from build123d import *

# Parameters (mm, degrees)
SKETCH1_W           = 203.2
SKETCH1_H           = 101.6
SKETCH1_R           = 1.27
SKETCH1_R_2         = 7.5184
SKETCH1_R_3         = 2.032
BOSS_EXTRUDE1_DEPTH = 3.175
SKETCH2_W           = 25.908
SKETCH2_H           = 3.175
CUT_EXTRUDE1_DEPTH  = 3.175
SKETCH3_W           = 25.908
SKETCH3_H           = 3.175
CUT_EXTRUDE2_DEPTH  = 3.175
SKETCH5_W           = 25.908
SKETCH5_H           = 3.175
CUT_EXTRUDE3_DEPTH  = 3.175
SKETCH6_W           = 25.908
SKETCH6_H           = 3.175
CUT_EXTRUDE4_DEPTH  = 3.175
SKETCH7_W           = 3.81
SKETCH7_H           = 19.558
CUT_EXTRUDE5_DEPTH  = 3.175


with BuildPart() as part:
    # Sketch1 → Boss-Extrude1 (new body)
    with BuildSketch(Plane(origin=(0, 0, 0), x_dir=(1, 0, 0), z_dir=(0, 1, 0))):
        with Locations((26.275862069, -0.437931034)):
            Rectangle(SKETCH1_W, SKETCH1_H)
        with Locations((120.357219561, 32.709068966)):
            Circle(SKETCH1_R, mode=Mode.SUBTRACT)
        with Locations((120.357219561, 42.869068966)):
            Circle(SKETCH1_R, mode=Mode.SUBTRACT)
        with Locations((-30.609137931, 35.837068966)):
            Circle(SKETCH1_R_2, mode=Mode.SUBTRACT)
        with Locations((-43.709137931, 35.837068966)):
            Circle(SKETCH1_R_3, mode=Mode.SUBTRACT)
        with Locations((-21.859137931, 44.737068966)):
            Circle(SKETCH1_R, mode=Mode.SUBTRACT)
        with Locations((-21.859137931, 26.937068966)):
            Circle(SKETCH1_R, mode=Mode.SUBTRACT)
    extrude(amount=BOSS_EXTRUDE1_DEPTH)

    # Sketch2 → Cut-Extrude1 (cut)
    with BuildSketch(Plane(origin=(0, 0, -50.362068966), x_dir=(-1, 0, 0), z_dir=(0, 0, -1))):
        with Locations((-89.775862069, 1.5875)):
            Rectangle(SKETCH2_W, SKETCH2_H)
        with Locations((-0.875862069, 1.5875)):
            Rectangle(SKETCH2_W, SKETCH2_H)
    extrude(amount=-CUT_EXTRUDE1_DEPTH, mode=Mode.SUBTRACT)

    # Sketch3 → Cut-Extrude2 (cut)
    with BuildSketch(Plane.XY.offset(51.237931034)):
        with Locations((0.875862069, 1.5875)):
            Rectangle(SKETCH3_W, SKETCH3_H)
        with Locations((89.775862069, 1.5875)):
            Rectangle(SKETCH3_W, SKETCH3_H)
    extrude(amount=-CUT_EXTRUDE2_DEPTH, mode=Mode.SUBTRACT)

    # Sketch5 → Cut-Extrude3 (cut)
    with BuildSketch(Plane.ZY.offset(75.324137931)):
        with Locations((0.437931034, 1.5875)):
            Rectangle(SKETCH5_W, SKETCH5_H)
    extrude(amount=-CUT_EXTRUDE3_DEPTH, mode=Mode.SUBTRACT)

    # Sketch6 → Cut-Extrude4 (cut)
    with BuildSketch(Plane(origin=(127.875862069, 0, 0), x_dir=(0, 0, -1), z_dir=(1, 0, 0))):
        with Locations((-0.437931034, 1.5875)):
            Rectangle(SKETCH6_W, SKETCH6_H)
    extrude(amount=-CUT_EXTRUDE4_DEPTH, mode=Mode.SUBTRACT)

    # Sketch7 → Cut-Extrude5 (cut)
    with BuildSketch(Plane.XZ):
        with Locations((125.970862069, -40.583068966)):
            Rectangle(SKETCH7_W, SKETCH7_H)
    extrude(amount=-CUT_EXTRUDE5_DEPTH, mode=Mode.SUBTRACT)


solid = part.part
The listing builds one solid part. Answer for the finished solid, in the listing's coordinates (mm). Round coordinates to 2 decimals unless told otherwise and drop trailing zeros. Loops run counter-clockwise (first coordinate to the right, second up) from the corner with the lowest first, then second, coordinate; pieces in that order, holes last. Notation, with made-up numbers: M 24,-16 L 54,-16 A30 cw 54,8 Z; hole C 3.25,72.5 d3. An arc over 180 degrees is marked long. Write each question's results on one line, items separated by ' | '. Start each with the question number.
1) Find section C-C on x = 11.5. Write down the section's boundary in (y, z) (3 decimals).
2) Straight lines are drawn through the part: probe 1 along Z at (x, y) = (-1.5, 0.5); probe 2 along X at (y, z) = (2.8, -10); probe 3 along Z at (x, y) = (-42, 2.2). For each, find the intervals that lie inside material, in ascending order.
3) Find section A-A on z = 11. Write down the section's boundary in (x, y) (3 decimals).
4) Determine the mould class of faces 1 (the flat face through (25, 0, 0)), 2 (the cylindrical face through (-31.59, 1.57, -43.29)) for opening direction Z: pulls with the +Z half, pulls with the -Z half, needs draft (parallel to the pull), parting line crosses it, or undercut.
5) Find section B-B on y = 0.9. Count the separate pieces of the cut face and the enclosed holes in it, plus the area to 3 significant figures.
6) Each of these flat-tipped pins is pushed along its axis until it touches: pin 1 (1 mm diameter, centred on y = 1.5, z = -48.5, fed in from +X); pin 2 (1.6 mm diameter, centred on x = -3.5, y = 2, fed in from +Z); pin 3 (1 mm diameter, centred on x = 126.5, y = 1.5, fed in from -Z); pin 4 (13.5 mm diameter, centred on x = -30.61, z = -35.84, fed in from +Y). Where does it stop, or does it pass through?
Final values:
1) outline: M 0,-47.187 L 3.175,-47.187 L 3.175,48.063 L 0,48.063 Z
2) probe 1: -47.19 to 48.06 | probe 2: -72.15 to 124.7 | probe 3: -50.36 to -36.94, -34.74 to 51.24
3) outline: M -72.149,0 L 124.701,0 L 124.701,3.175 L -72.149,3.175 Z
4) face 1: needs draft | face 2: undercut
5) separate pieces: 1 | enclosed holes: 6 | area: 19,900 mm²
6) pin 1: x = 124.07 | pin 2: z = 48.06 | pin 3: z = -30.8 | pin 4: through
